Check sheet for the drawn part. Datum: minimum x, y, z corner. Units: mm. Coordinates: 2 decimals unless noted, no trailing zeros. Write each loop counter-clockwise with the first axis right and the second up, starting at its lowest first coordinate (ties: lowest second). Pieces come first, ordered by that corner, then holes. Notation, with made-up numbers: M 77.5,-15 L 136.5,-15 A10 ccw 136.5,3 Z; hole C -28,-27 d9. An arc over 180 degrees is marked long. Answer as CSV lines item,"result". Start each with the question number.
Q1. Thickness scan on line 1 along Y through (x, z) = (10, 1.9); line 2 along X through (y, z) = (5.75, 4); line 3 along Z through (x, y) = (18.5, 11.5). Record the ranges inside material, lowest first. Write a range as from..to.
Q2. Sectioned sample at A-A, the plane y = 10. Record the cut outline in (x, z), then the cut area to 3 significant figures.
Q3. Sectioned sample at D-D, the plane z = 2.5. Record the cut outline in (x, y).
Q4. Sectioned sample at B-B, the plane z = 5.25. Record the cut outline in (x, y), then the cut area to 3 significant figures.
Q5. Mould release check, pull along X, two halves, no side actions. Record for the marked faces 1, 2 and 3: pulls with the +X half, pulls with the -X half, needs draft (parallel to the pull), parting line crosses it, or undercut.
Q6. Depth check by flat-ended pin: pin 1 Ø10 at (x, y) = (3.5, 13) entering from -Z; pin 2 Ø0.6 at (y, z) = (10.5, 5.5) entering from +X; pin 3 Ø0.5 at (x, z) = (1, 5.5) entering from +Y; pin 4 Ø2 at (x, y) = (18, 3.5) entering from +Z. Enter the tip coordinate at first touch or a pass-through.
Q7. Sectioned sample at C-C, the plane x = 8. Record the cut outline in (y, z).
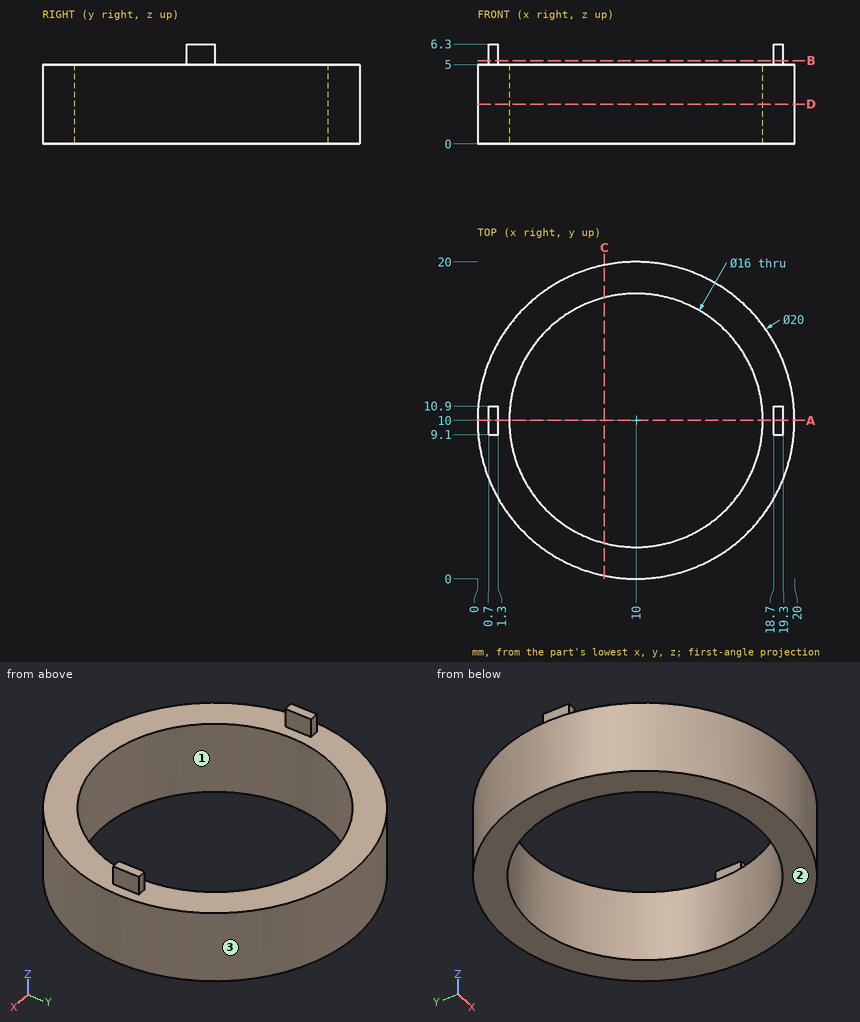
Output:
1,line 1,"y = 0..2, 18..20"
1,line 2,"x = 0.95..3.22, 16.78..19.05"
1,line 3,"z = 0..5"
2,outline,"M 0,0 L 2,0 L 2,5 L 1.3,5 L 1.3,6.3 L 0.7,6.3 L 0.7,5 L 0,5 Z; M 18,0 L 20,0 L 20,5 L 19.3,5 L 19.3,6.3 L 18.7,6.3 L 18.7,5 L 18,5 Z"
2,area,"21.6 mm^2"
3,outline,"C 10,10 d20; hole C 10,10 d16"
4,outline,"M 0.7,9.1 L 1.3,9.1 L 1.3,10.9 L 0.7,10.9 Z; M 18.7,9.1 L 19.3,9.1 L 19.3,10.9 L 18.7,10.9 Z"
4,area,"2.16 mm^2"
5,face 1,"undercut"
5,face 2,"needs draft"
5,face 3,"parting line crosses it"
6,pin 1,"stops at z = 0"
6,pin 2,"stops at x = 19.3"
6,pin 3,"stops at y = 10.9"
6,pin 4,"stops at z = 5"
7,outline,"M 0.2,0 L 2.25,0 L 2.25,5 L 0.2,5 Z; M 17.75,0 L 19.8,0 L 19.8,5 L 17.75,5 Z"
